CAD build for the part. Positions are in the model's coordinates, mm. Face numbers are marked on the shaded views. Round coordinates to 2 decimals unless told otherwise and drop trailing zeros. Loops run counter-clockwise (first coordinate to the right, second up) from the corner with the lowest first, then second, coordinate; pieces in that order, holes last.
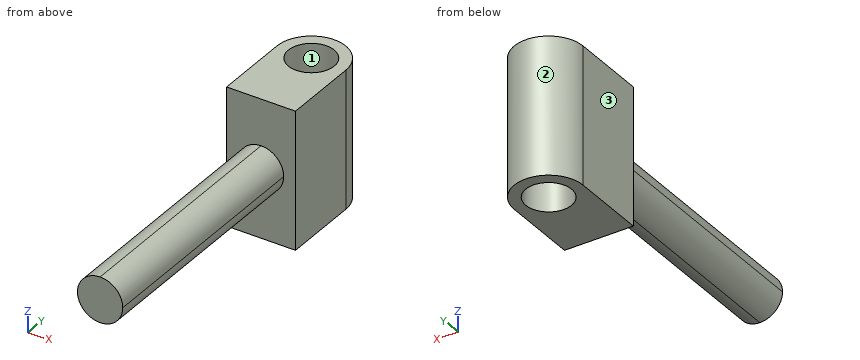
from build123d import *

# Parameters (mm, degrees)
BOSS_EXTRUDE1_DEPTH = 45.72
SKETCH2_R           = 7.62
CUT_EXTRUDE1_DEPTH  = 10.414
SKETCH3_R           = 7.62
CUT_EXTRUDE2_DEPTH  = 76.2
BOSS_EXTRUDE2_DEPTH = 81.28


with BuildPart() as part:
    # Sketch1 → Boss-Extrude1 (new body)
    with BuildSketch(Plane.XY):
        with BuildLine():
            Line((-11.43, 0), (-11.43, -25.4))
            Line((-11.43, -25.4), (11.43, -25.4))
            Line((11.43, -25.4), (11.43, 0))
            ThreePointArc((11.43, 0), (0, 11.43), (-11.43, 0))
        make_face()
    extrude(amount=BOSS_EXTRUDE1_DEPTH)

    # Sketch2 → Cut-Extrude1 (cut)
    with BuildSketch(Plane.XY.offset(45.72)):
        Circle(SKETCH2_R)
    extrude(amount=-CUT_EXTRUDE1_DEPTH, mode=Mode.SUBTRACT)

    # Sketch3 → Cut-Extrude2 (cut)
    with BuildSketch(Plane.XY.offset(45.72)):
        Circle(SKETCH3_R)
    extrude(amount=-CUT_EXTRUDE2_DEPTH, mode=Mode.SUBTRACT)

    # Sketch4 → Boss-Extrude2 (add)
    with BuildSketch(Plane.XZ.offset(25.4)):
        with BuildLine():
            ThreePointArc((-7.514066823, 22.86), (-5.313247605, 17.546752395), (0, 15.345933177))
            Line((0, 15.345933177), (0, 22.86))
            Line((0, 22.86), (-7.514066823, 22.86))
        make_face()
        with BuildLine():
            Line((0, 22.86), (0, 15.345933177))
            ThreePointArc((0, 15.345933177), (5.313247605, 17.546752395), (7.514066823, 22.86))
            Line((7.514066823, 22.86), (0, 22.86))
        make_face()
        with BuildLine():
            Line((-7.514066823, 22.86), (0, 22.86))
            Line((0, 22.86), (0, 30.374066823))
            ThreePointArc((0, 30.374066823), (-5.313247605, 28.173247605), (-7.514066823, 22.86))
        make_face()
        with BuildLine():
            Line((0, 30.374066823), (0, 22.86))
            Line((0, 22.86), (7.514066823, 22.86))
            ThreePointArc((7.514066823, 22.86), (5.313247605, 28.173247605), (0, 30.374066823))
        make_face()
    extrude(amount=BOSS_EXTRUDE2_DEPTH)


solid = part.part
Item 1: Cut at A-A (z = 35). List the corners of the cut face in (x, y).
Verdict:
outline: (-11.43, -25.4) - (11.43, -25.4) - (11.43, 0) arc R11.43 ccw to (-11.43, 0) - close; hole circle Ø15.24 at (0, 0)
Item 2: Flat gauge pins, fed straight in: P1, Ø8, axis at y = -41.5, z = 12, coming from the +X side; P2, Ø12, axis at y = -79, z = 28, coming from the -X side; P3, Ø1, axis at x = 7.5, z = 28.5, coming from the -Y side. Where does each tip first touch, or does it go through?
Verdict:
P1: stops at x = 3.07
P2: stops at x = -7.51
P3: stops at y = -25.4
Item 3: Cut at C-C (y = 2). List the corners of the cut face in (x, z), plus the area to 3 significant figures.
Verdict:
outline: (-11.25, 0) - (-7.35, 0) - (-7.35, 45.72) - (-11.25, 45.72) - close; (7.35, 0) - (11.25, 0) - (11.25, 45.72) - (7.35, 45.72) - close
area: 357 mm2
Item 4: Wall check: L1, parallel to Y at x = 0, z = 12; L2, parallel to Y at x = -6.75, z = 32; L3, parallel to Y at x = 8, z = 21. Give the ranges that are in metal, low to high.
Verdict:
L1: y = -25.4 to -7.62, 7.62 to 11.43
L2: y = -25.4 to -3.54, 3.54 to 9.22
L3: y = -25.4 to 8.16
Item 5: Cut at B-B (x = 5.5). List the corners of the cut face in (y, z), plus the area to 3 significant figures.
Verdict:
outline: (-106.68, 17.74) - (-25.4, 17.74) - (-25.4, 0) - (-5.27, 0) - (-5.27, 45.72) - (-25.4, 45.72) - (-25.4, 27.98) - (-106.68, 27.98) - close; (5.27, 0) - (10.02, 0) - (10.02, 45.72) - (5.27, 45.72) - close
area: 1,970 mm2
Item 6: Cut at D-D (y = -49). List the corners of the cut face in (x, z), plus the area to 3 significant figures.
Verdict:
outline: circle Ø15.03 at (0, 22.86)
area: 177 mm2
Item 7: Mould opens along X. For the marked faces 1, 2 and 3 say: released by +X, released by -X, zero draft, split by the parting line, or undercut.
Verdict:
face 1: undercut
face 2: split by the parting line
face 3: released by -X
